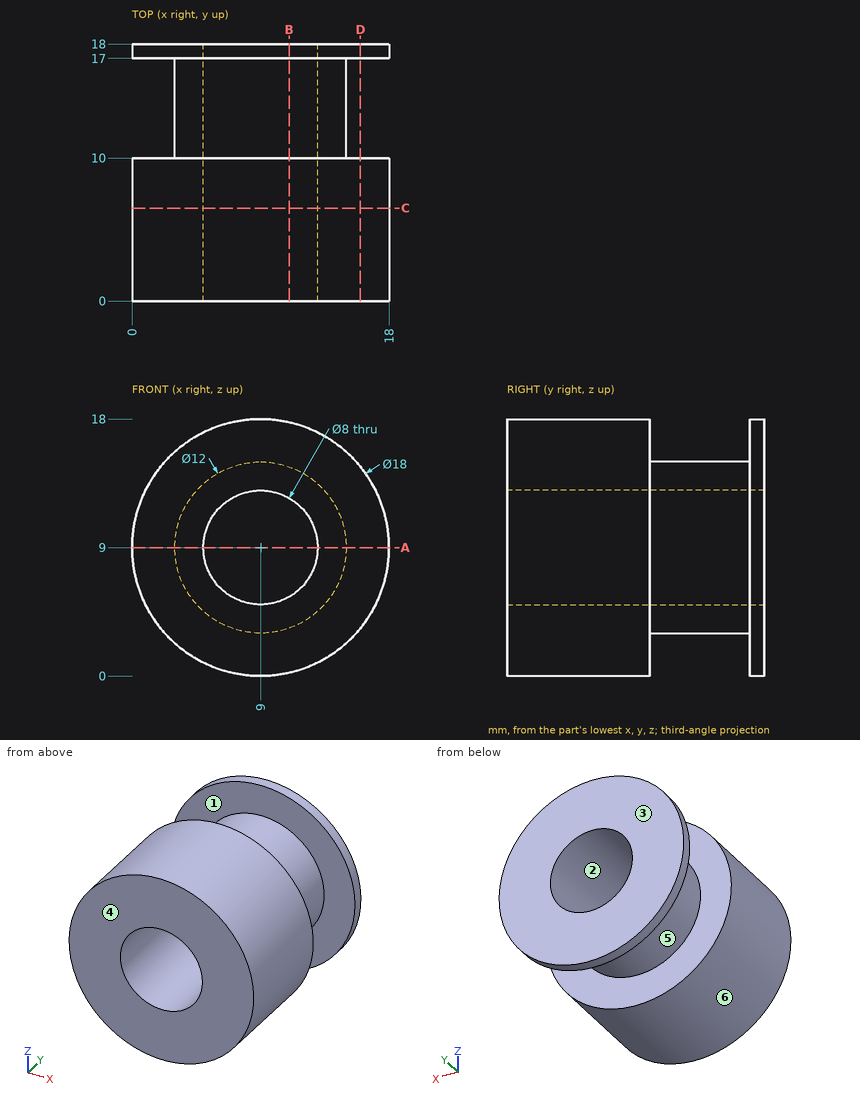
Design review of the part shown in the three views and the two pictorial views. Dimensions are in mm from the part's minimum x, y and z. A direction names the side the tool comes from. Coordinates: 2 decimals unless noted, no trailing zeros. Order: outer loops, then holes, each group sorted by start corner. A loop starts at its lowest first (then second) coordinate and runs counter-clockwise, first axis right, second up.
Item 1: Take a section at C-C, the plane y = 6.5. Write out the cut boundary in (x, z).
Item 2: For the marked faces 5 and 6, list the 3-axis set-ups (+Z, -Z, +X, -X, +Y, -Y) from which the entire face can be reached by the end or side of a thin tool; tool diameter is ignored.
Item 3: For pin 1 Ø3 at (y, z) = (13.5, 13) entering from +X; pin 2 Ø1.5 at (x, y) = (6, 7) entering from +Z; pin 3 Ø4 at (y, z) = (13, 7.5) entering from -X, all flat-tipped, find the tip position at first contact; note any pin that passes through.
Item 4: Take a section at A-A, the plane z = 9. Write out the cut boundary in (x, y), then the cut area to 3 significant figures.
Item 5: Take a section at B-B, the plane x = 11. Write out the cut boundary in (y, z), then the cut area to 3 significant figures.
Item 6: For line 1 (Y direction, x = 16, z = 6.5); line 2 (X direction, y = 4.75, z = 9); line 3 (X direction, y = 11.25, z = 9), list the stretches that pass through material, from the lowest coordinate up.
Item 7: The part is to be moulded in two halves that separate along Y. For the marked faces 1, 2, 3 and 4, say which applies: pulls with the +Y half, pulls with the -Y half, needs draft (parallel to the pull), parting line crosses it, or undercut.
Item 8: Take a section at D-D, the plane x = 16. Write out the cut boundary in (y, z).
The answers:
1. outline: circle Ø18 at (9, 9); hole circle Ø8 at (9, 9)
2. face 5: none
2. face 6: +Y, -Y
3. pin 1: stops at x = 14.45
3. pin 2: stops at z = 17.71
3. pin 3: stops at x = 3
4. outline: (0, 0) - (5, 0) - (5, 18) - (0, 18) - (0, 17) - (3, 17) - (3, 10) - (0, 10) - close; (13, 0) - (18, 0) - (18, 10) - (15, 10) - (15, 17) - (18, 17) - (18, 18) - (13, 18) - close
4. area: 138 mm2
5. outline: (0, 0.23) - (10, 0.23) - (10, 3.34) - (17, 3.34) - (17, 0.23) - (18, 0.23) - (18, 5.54) - (0, 5.54) - close; (0, 12.46) - (18, 12.46) - (18, 17.77) - (17, 17.77) - (17, 14.66) - (10, 14.66) - (10, 17.77) - (0, 17.77) - close
5. area: 148 mm2
6. line 1: y = 0 to 10, 17 to 18
6. line 2: x = 0 to 5, 13 to 18
6. line 3: x = 3 to 5, 13 to 15
7. face 1: undercut
7. face 2: needs draft
7. face 3: pulls with the +Y half
7. face 4: pulls with the -Y half
8. outline: (0, 3.34) - (10, 3.34) - (10, 14.66) - (0, 14.66) - close; (17, 3.34) - (18, 3.34) - (18, 14.66) - (17, 14.66) - close
